Build history of the part. All positions in model axes, mm. A direction names the side the tool comes from. Round coordinates to 2 decimals unless told otherwise and drop trailing zeros. Order: outer loops, then holes, each group sorted by start corner. A loop starts at its lowest first (then second) coordinate and runs counter-clockwise, first axis right, second up. Notation, with made-up numbers: M -13,25.5 L 44,25.5 A21 ccw 44,45.5 Z; hole C 10,54 d9. An arc over 180 degrees is marked long. Use CSV: the item, a comma, the result in double quotes.
from build123d import *

# Parameters (mm, degrees)
SKETCH1_W           = 15.24
SKETCH1_H           = 136.915
BOSS_EXTRUDE1_DEPTH = 10
SKETCH2_R           = 5.3
CUT_EXTRUDE1_DEPTH  = 165.72630229
BOSS_EXTRUDE2_DEPTH = 15.24
BOSS_EXTRUDE3_DEPTH = 10
FILLET7_R           = 7.62
FILLET8_R           = 7.62


with BuildPart() as part:
    # Sketch1 → Boss-Extrude1 (new body)
    with BuildSketch(Plane(origin=(37.730745885, 0, 0), x_dir=(0, 0, -1), z_dir=(1, 0, 0))):
        with Locations((136.328078847, -11.001327465)):
            Rectangle(SKETCH1_W, SKETCH1_H)
    extrude(amount=BOSS_EXTRUDE1_DEPTH)

    # Sketch2 → Cut-Extrude1 (cut, through all)
    with BuildSketch(Plane(origin=(47.730745885, 0, 0), x_dir=(0, 0, -1), z_dir=(1, 0, 0))):
        with Locations((136.328078847, 49.836172535)):
            Circle(SKETCH2_R)
    extrude(amount=-CUT_EXTRUDE1_DEPTH, mode=Mode.SUBTRACT)

    # Sketch4 → Boss-Extrude2 (add)
    with BuildSketch(Plane(origin=(0, 0, -143.948078847), x_dir=(-1, 0, 0), z_dir=(0, 0, -1))):
        Polygon((-37.730745885, -79.458827465), (-5.980745885, -79.458827465), (-37.730745885, -54.058827465), align=None)
    extrude(amount=-BOSS_EXTRUDE2_DEPTH)

    # Sketch6 → Boss-Extrude3 (add)
    with BuildSketch(Plane(origin=(47.730745885, 0, 0), x_dir=(0, 0, -1), z_dir=(1, 0, 0))):
        Polygon((128.708078847, -79.458827465), (116.008078847, -79.458827465), (89.258078847, -79.458827465), (89.258078847, -69.458827465), (121.008078847, -69.458827465), (128.708078847, -54.058827465), align=None)
    extrude(amount=-BOSS_EXTRUDE3_DEPTH)

    # Fillet7
    # the kernel refuses this fillet: 7.62 mm, written as the material it adds along each edge
    with BuildSketch(Plane(origin=(37.730745885, -54.058827465, -143.948078847), x_dir=(-0.7808688094430346, -0.6246950475544188, 2.599749935093665e-15), z_dir=(0, 0, 1))) as fillet7_piece_1:
        with BuildLine():
            CenterArc((FILLET7_R * 0.480624847487, -FILLET7_R), FILLET7_R, 90, 51.340191746)
            Line((-FILLET7_R * 0.300243961956, -FILLET7_R * 0.375304952446), (0, 0))
            Line((0, 0), (FILLET7_R * 0.480624847487, 0))
        make_face()
    extrude(amount=15.24)
    with BuildSketch(Plane(origin=(47.730745885, -69.458827465, -121.008078847), x_dir=(-1.4253394908736166e-15, 0.8944271909999135, -0.4472135954999628), z_dir=(-1, 0, 0))) as fillet7_piece_2:
        with BuildLine():
            CenterArc((FILLET7_R * 0.61803398875, -FILLET7_R), FILLET7_R, 90, 63.434948823)
            Line((-FILLET7_R * 0.27639320225, -FILLET7_R * 0.5527864045), (0, 0))
            Line((0, 0), (FILLET7_R * 0.61803398875, 0))
        make_face()
    extrude(amount=10)

    # Fillet8
    fillet8_edges = [part.edges().sort_by_distance(p)[0] for p in [
        (42.730745885, -54.058827465, -128.708078847),
    ]]
    fillet(fillet8_edges, radius=FILLET8_R)


solid = part.part
(1) Cut at A-A, the plane z = -136. Give the cut face in (x, y).
Answer block:
outline,"M 5.98,-79.46 L 47.73,-79.46 L 47.73,44.55 L 37.73,44.55 L 37.73,-50.4 A7.62 cw 34.87,-56.35 Z; M 37.73,55.13 L 47.73,55.13 L 47.73,57.46 L 37.73,57.46 Z"
(2) Cut at B-B, the plane y = -30.5. Give the cut face in (x, z).
Answer block:
outline,"M 37.73,-143.95 L 47.73,-143.95 L 47.73,-128.71 L 37.73,-128.71 Z"
(3) Cut at D-D, the plane z = -121.5. Give the cut face in (x, y).
Answer block:
outline,"M 37.73,-79.46 L 47.73,-79.46 L 47.73,-67.41 L 37.73,-67.41 Z"
(4) Two-plate mould, pull along Y, no slides. Class faces 1 (the face through (43, 57.456, -136)), 2 (the face through (47.731, -25, -133)), 3 (the face through (42.801, 51.428, -141.383)): released by +Y, released by -Y, zero draft, split by the parting line, or undercut.
Answer block:
face 1,"released by +Y"
face 2,"zero draft"
face 3,"undercut"
(5) Wall check: line 1 (X direction, y = -36.5, z = -133); line 2 (Y direction, x = 41, z = -133); line 3 (Z direction, x = 38, y = 52). Give the ranges that are in metal, low to high. Write a range as from..to.
Answer block:
line 1,"x = 37.73..47.73"
line 2,"y = -79.46..45.71, 53.96..57.46"
line 3,"z = -143.95..-141.17, -131.49..-128.71"
(6) Tool access for faces 4 (the face through (37.731, -72, -112)), 5 (the face through (43, -69.459, -103)), 6 (the face through (40, -14, -128.708)), 7 (the face through (37.731, 4, -136)): list every direction of +Z, -Z, +X, -X, +Y, -Y with a clear straight run to the whole face (end or side of a thin tool).
Answer block:
face 4,"+Z, -X, +Y, -Y"
face 5,"+Z, +X, -X, +Y"
face 6,"+Z, -X, +Y"
face 7,"+Z, -Z, -X, +Y"
(7) Cut at C-C, the plane x = 42. Give the cut face in (y, z), and give its area (3 significant figures).
Answer block:
outline,"M -79.46,-143.95 L 57.46,-143.95 L 57.46,-128.71 L -52.26,-128.71 A7.62 cw -55.67,-127.9 L -65.25,-123.11 A7.62 cw -69.46,-116.3 L -69.46,-89.26 L -79.46,-89.26 Z; hole C 49.84,-136.33 d10.6"
area,"2,460 mm²"
(8) Drop flat-ended pins along their axis: pin 1 (5 mm diameter, centred on x = 22.5, z = -138, fed in from +Y); pin 2 (12 mm diameter, centred on x = 36.5, z = -105, fed in from +Y); pin 3 (4.5 mm diameter, centred on y = 21.5, z = -133.5, fed in from -X). Give the stop position or say it passes through.
Answer block:
pin 1,"stops at y = -64.24"
pin 2,"stops at y = -69.46"
pin 3,"stops at x = 37.73"
